Part print with two shaded views. Sizes in mm from the minimum x, y, z corner. A direction names the side the tool comes from. Give positions to 0.01 mm unless a question says otherwise; leave off trailing zeros. Loops run counter-clockwise (first coordinate to the right, second up) from the corner with the lowest first, then second, coordinate; pieces in that order, holes last. Notation, with made-up numbers: M 84,28.5 L 135,28.5 A21 ccw 135,54.5 Z; hole C 87,41.25 d5. An arc over 180 degrees is marked long. Answer in a Markdown table with one row per item.
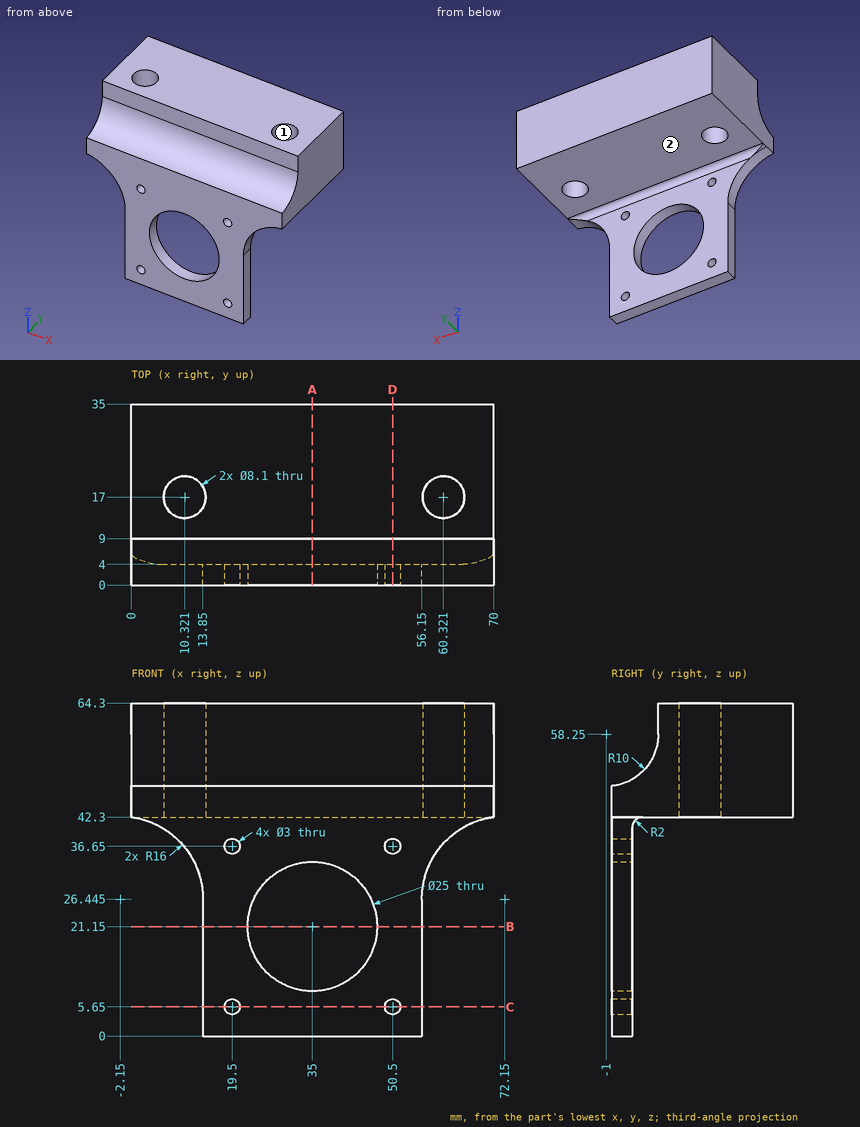
Q1. 3-axis set-ups, long thin cutter, end or side, ignore diameter. For the marked faces 1 and 2: which of +Z, -Z, +X, -X, +Y, -Y reach the whole face in a straight line?
Reported:
| item | result |
|---|---|
| face 1 | +Z, -Z |
| face 2 | -Z, +X, -X, +Y |
Q2. Drop flat-ended pins along their axis: pin 1 (14.5 mm diameter, centred on x = 32, y = 25, fed in from -Z); pin 2 (6.5 mm diameter, centred on x = 26.5, z = 61.5, fed in from -Y); pin 3 (4.5 mm diameter, centred on y = 2, z = 10, fed in from -X). Give the stop position or say it passes through.
Reported:
| item | result |
|---|---|
| pin 1 | z = 42.3 |
| pin 2 | y = 9 |
| pin 3 | x = 13.85 |
Q3. Saw through at B-B (z = 21.15). Give the cut face in (x, y).
Reported:
| item | result |
|---|---|
| outline | M 13.85,0 L 22.5,0 L 22.5,4 L 13.85,4 Z; M 47.5,0 L 56.15,0 L 56.15,4 L 47.5,4 Z |
Q4. Saw through at C-C (z = 5.65). Give the cut face in (x, y).
Reported:
| item | result |
|---|---|
| outline | M 13.85,0 L 18,0 L 18,4 L 13.85,4 Z; M 21,0 L 49,0 L 49,4 L 21,4 Z; M 52,0 L 56.15,0 L 56.15,4 L 52,4 Z |
Q5. Saw through at D-D (x = 50.5). Give the cut face in (y, z), and give its area (3 significant figures).
Reported:
| item | result |
|---|---|
| outline | M 0,0 L 4,0 L 4,4.15 L 0,4.15 Z; M 0,7.15 L 4,7.15 L 4,35.15 L 0,35.15 Z; M 0,38.15 L 4,38.15 L 4,40.3 A2 cw 6,42.3 L 35,42.3 L 35,64.3 L 9,64.3 L 9,58.25 A10 cw 0,48.3 Z |
| area | 793 mm² |
Q6. Probe probe 1 along Z at (x, y) = (34.5, 32.5); probe 2 along X at (y, z) = (1.05, 21.15); probe 3 along X at (y, z) = (2, 36). List the from-to ranges inside material, lowest first.
Reported:
| item | result |
|---|---|
| probe 1 | 42.3 to 64.3 |
| probe 2 | 13.85 to 22.5, 47.5 to 56.15 |
| probe 3 | 10.68 to 18.15, 20.85 to 49.15, 51.85 to 59.32 |
Q7. Saw through at A-A (x = 35). Give the cut face in (y, z).
Reported:
| item | result |
|---|---|
| outline | M 0,0 L 4,0 L 4,8.65 L 0,8.65 Z; M 0,33.65 L 4,33.65 L 4,40.3 A2 cw 6,42.3 L 35,42.3 L 35,64.3 L 9,64.3 L 9,58.25 A10 cw 0,48.3 Z |
